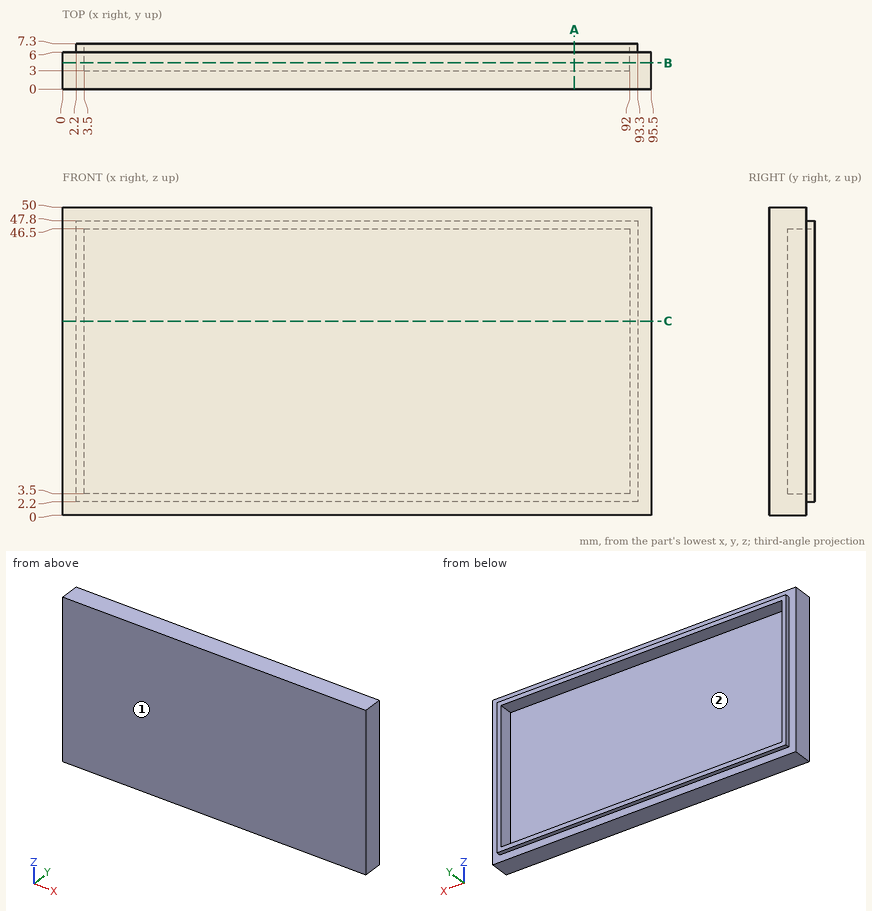
Input: dimensioned drawing with shaded views. Units: mm. Origin: part minimum x, y, z. Round coordinates to 2 decimals unless told otherwise and drop trailing zeros. Order: outer loops, then holes, each group sorted by start corner. A loop starts at its lowest first (then second) coordinate and runs counter-clockwise, first axis right, second up. Notation, with made-up numbers: M -20,83 L 10,83 A29 ccw 10,121 Z; hole C 7.25,27 d7. An arc over 180 degrees is marked long. Use one line per item in the form item = value. Start each with the question number.
Q1. Mould query, pull axis X, two halves, no side actions, for the marked faces 1 and 2. Classes: +X half, -X half, draft (parallel to the pull), parting line (faces both ways), or undercut.
Q2. Cut plane C-C (z = 31.5). Return loops of the section in (x, y), and give its area (3 significant figures).
Q3. Material intervals for line 1 (Z direction, x = 66, y = 4.5); line 2 (X direction, y = 5.75, z = 33); line 3 (X direction, y = 7, z = 41), sorted ascending. Write a range as [from, to].
Q4. Pin query (flat end, axial travel): pin 1 Ø5 at (x, z) = (24, 33) entering from +Y; pin 2 Ø0.6 at (x, y) = (63.5, 6.5) entering from -Z; pin 3 Ø0.6 at (x, y) = (59, 6.5) entering from +Z. Return the tip coordinate at first contact, or that it passes through.
Q5. Cut plane B-B (y = 4.25). Return loops of the section in (x, z), and give its area (4 significant figures).
Q6. Cut plane A-A (x = 83). Return loops of the section in (y, z).
Geometry results:
q1.face_1 = draft
q1.face_2 = undercut
q2.outline = M 0,0 L 95.5,0 L 95.5,6 L 93.3,6 L 93.3,7.3 L 92,7.3 L 92,3 L 3.5,3 L 3.5,7.3 L 2.2,7.3 L 2.2,6 L 0,6 Z
q2.area = 311 mm^2
q3.line_1 = [0, 3.5], [46.5, 50]
q3.line_2 = [0, 3.5], [92, 95.5]
q3.line_3 = [2.2, 3.5], [92, 93.3]
q4.pin_1 = 3
q4.pin_2 = 2.2
q4.pin_3 = 47.8
q5.outline = M 0,0 L 95.5,0 L 95.5,50 L 0,50 Z; hole M 3.5,3.5 L 92,3.5 L 92,46.5 L 3.5,46.5 Z
q5.area = 969.5 mm^2
q6.outline = M 0,0 L 6,0 L 6,2.2 L 7.3,2.2 L 7.3,3.5 L 3,3.5 L 3,46.5 L 7.3,46.5 L 7.3,47.8 L 6,47.8 L 6,50 L 0,50 Z
